```python
from build123d import *

# Parameters (mm, degrees)
F0_W     = 105
F0_H     = 110
F1_DEPTH = 90
F2_T     = -2.5
F3_R     = 5.1
F3_R_2   = 5
F4_DEPTH = 25


with BuildPart() as f1:
    # F0 (on Front) → F1 (new body)
    with BuildSketch(Plane.XZ):
        Rectangle(F0_W, F0_H)
    extrude(amount=F1_DEPTH)

    # F2
    f2_openings = [f1.faces().sort_by_distance(p)[0] for p in [
        (0, -90, 0),
    ]]
    offset(amount=F2_T, openings=f2_openings)

    # F3 (on face) → F4 (cut)
    with BuildSketch(Plane.XY.offset(55)):
        with Locations((16.6, -51.43)):
            Circle(F3_R)
        with Locations((33, -80)):
            Circle(F3_R)
        with Locations((0, -80)):
            Circle(F3_R)
        with Locations((-33, -80)):
            Circle(F3_R)
        with Locations((-16.5, -51.43)):
            Circle(F3_R)
        with Locations((0, -22.86)):
            Circle(F3_R_2)
    extrude(amount=-F4_DEPTH, mode=Mode.SUBTRACT)


solid = f1.part
```
The model under review builds one solid part; all positions refer to its coordinate system, in mm. A direction names the side the tool comes from. Give positions to 0.01 mm unless a question says otherwise; leave off trailing zeros. Loops run counter-clockwise (first coordinate to the right, second up) from the corner with the lowest first, then second, coordinate; pieces in that order, holes last. Notation, with made-up numbers: (-4, -19.75) -> (27, -19.75) arc R8 ccw to (27, -9.75) -> close; hole circle Ø11 at (79.25, 32). An arc over 180 degrees is marked (long way). Use CSV: the item, a comma, the result in double quotes.
1. Consider section C-C, the plane y = -41. Write out the cut boundary in (x, z), then the cut area to 3 significant figures.
Result:
outline,"(-52.5, -55) -> (52.5, -55) -> (52.5, 55) -> (-52.5, 55) -> close; hole (-50, -52.5) -> (50, -52.5) -> (50, 52.5) -> (-50, 52.5) -> close"
area,"1,050 mm²"
2. Machinability: for faces 4 (the face through (-1, -75, 54)), 5 (the face through (-1, 0, 1)), 6 (the face through (-1, -46, -52.5)), which of the approach directions +Z, -Z, +X, -X, +Y, -Y give a long, thin tool a straight path to every point of the face, cutting with its end or side? Answer none if there is none.
Result:
face 4,"+Z"
face 5,"+Z, -Z, +X, -X, +Y"
face 6,"-Y"
3. For P1, Ø12, axis at x = 31.5, z = 16, coming from the -Y side, flat-tipped, find the tip position at first contact; note if it passes through.
Result:
P1,"stops at y = -2.5"
4. To check wall thickness, follow probe 1 along Y at (x, z) = (0, 53); probe 2 along X at (y, z) = (-51, 53); probe 3 along X at (y, z) = (-36, -24). State the ranges of each line that lie inside material, in increasing order. Write a range as from..to.
Result:
probe 1,"y = -90..-85.1, -74.9..-27.86, -17.86..0"
probe 2,"x = -52.5..-21.58, -11.42..11.52, 21.68..52.5"
probe 3,"x = -52.5..-50, 50..52.5"
5. Consider section A-A, the plane x = 33. Write out the cut boundary in (y, z), then the cut area to 3 significant figures.
Result:
outline,"(-90, -55) -> (0, -55) -> (0, 55) -> (-74.9, 55) -> (-74.9, 52.5) -> (-2.5, 52.5) -> (-2.5, -52.5) -> (-90, -52.5) -> close; (-90, 52.5) -> (-85.1, 52.5) -> (-85.1, 55) -> (-90, 55) -> close"
area,"687 mm²"
6. Consider section B-B, the plane y = -51.43. Write out the cut boundary in (x, z).
Result:
outline,"(-52.5, -55) -> (52.5, -55) -> (52.5, 55) -> (21.7, 55) -> (21.7, 52.5) -> (50, 52.5) -> (50, -52.5) -> (-50, -52.5) -> (-50, 52.5) -> (-21.6, 52.5) -> (-21.6, 55) -> (-52.5, 55) -> close; (-11.4, 52.5) -> (11.5, 52.5) -> (11.5, 55) -> (-11.4, 55) -> close"
7. Consider section D-D, the plane x = 0. Write out the cut boundary in (y, z), then the cut area to 3 significant figures.
Result:
outline,"(-90, -55) -> (0, -55) -> (0, 55) -> (-17.86, 55) -> (-17.86, 52.5) -> (-2.5, 52.5) -> (-2.5, -52.5) -> (-90, -52.5) -> close; (-90, 52.5) -> (-85.1, 52.5) -> (-85.1, 55) -> (-90, 55) -> close; (-74.9, 52.5) -> (-27.86, 52.5) -> (-27.86, 55) -> (-74.9, 55) -> close"
area,"662 mm²"
8. The part is to be moulded in two halves that separate along Z. For faces 1 (the face through (-50, -46, -1)), 2 (the face through (29.2, -76.6, 53.8)), 3 (the face through (-1, -44, -55)), say which applies: +Z half, -Z half, draft (parallel to the pull), parting line (faces both ways), or undercut.
Result:
face 1,"undercut"
face 2,"draft"
face 3,"-Z half"
